Geometry check sheet. Reference: the model listing, model coordinates, mm. A direction names the side the tool comes from. Give positions to 0.01 mm unless a question says otherwise; leave off trailing zeros. Write each loop counter-clockwise with the first axis right and the second up, starting at its lowest first coordinate (ties: lowest second). Pieces come first, ordered by that corner, then holes. Notation, with made-up numbers: (40, 78.25) -> (87, 78.25) arc R5 ccw to (87, 83.25) -> close; hole circle Ø9 at (-5, 6). An arc over 180 degrees is marked (long way). One line per item, written item: value.
from build123d import *

# Parameters (mm, degrees)
BOSS_EXTRUDE1_DEPTH = 6.8
SKETCH2_W           = 3.55
SKETCH2_H           = 7.5
SKETCH2_W_2         = 2.085
SKETCH2_H_2         = 5
SKETCH2_H_3         = 8.5
CUT_EXTRUDE1_DEPTH  = 6.8
SKETCH3_R           = 6.1
CUT_EXTRUDE2_DEPTH  = 6.8
SKETCH4_R           = 1.75
CUT_EXTRUDE3_DEPTH  = 6.8


with BuildPart() as part:
    # Sketch1 → Boss-Extrude1 (new body)
    with BuildSketch(Plane.XY):
        with BuildLine():
            Line((-97, 195.4), (-92.5, 195.4))
            Line((-92.5, 195.4), (-92.5, 170.4))
            Line((-92.5, 170.4), (-89.2, 170.4))
            Line((-89.2, 170.4), (-89.2, 168.4))
            Line((-89.2, 168.4), (-82.3, 168.4))
            Line((-82.3, 168.4), (-82.3, 170.4))
            Line((-82.3, 170.4), (-79, 170.4))
            Line((-79, 170.4), (-79, 195.4))
            Line((-79, 195.4), (-75.034597787, 195.4))
            ThreePointArc((-75.034597787, 195.4), (-71.177872129, 193.996266659), (-69.125751269, 190.441889066))
            Line((-69.125751269, 190.441889066), (-64.181209637, 162.4))
            ThreePointArc((-64.181209637, 162.4), (-55.56310459, 141.196422986), (-39, 125.4))
            ThreePointArc((-39, 125.4), (-10.413345727, 95.649656796), (0, 55.726706578))
            Line((0, 55.726706578), (0, 0))
            Line((0, 0), (-78, 0))
            Line((-78, 0), (-78, 64.670637847))
            ThreePointArc((-78, 64.670637847), (-82.987756652, 97.72473667), (-97.652405773, 127.764697248))
            ThreePointArc((-97.652405773, 127.764697248), (-101.631906793, 135.904056195), (-103, 144.860278245))
            Line((-103, 144.860278245), (-103, 189.4))
            ThreePointArc((-103, 189.4), (-101.242640687, 193.642640687), (-97, 195.4))
        make_face()
    extrude(amount=BOSS_EXTRUDE1_DEPTH)

    # Sketch2 → Cut-Extrude1 (cut)
    with BuildSketch(Plane.XY.offset(6.8)):
        with Locations((-19, 17.25)):
            Rectangle(SKETCH2_W, SKETCH2_H)
        with Locations((-21.8175, 11)):
            Rectangle(SKETCH2_W_2, SKETCH2_H_2)
        with Locations((-16.1825, 11)):
            Rectangle(SKETCH2_W_2, SKETCH2_H_2)
        with Locations((-19, 4.25)):
            Rectangle(SKETCH2_W, SKETCH2_H_3)
        with Locations((-19, 11)):
            Rectangle(SKETCH2_W, SKETCH2_H_2)
    extrude(amount=-CUT_EXTRUDE1_DEPTH, mode=Mode.SUBTRACT)

    # Sketch3 → Cut-Extrude2 (cut)
    with BuildSketch(Plane.XY.offset(6.8)):
        with Locations((-59.04, -1.33811552)):
            Circle(SKETCH3_R)
    extrude(amount=-CUT_EXTRUDE2_DEPTH, mode=Mode.SUBTRACT)

    # Sketch4 → Cut-Extrude3 (cut)
    with BuildSketch(Plane(origin=(0, 0, 0), x_dir=(-1, 0, 0), z_dir=(0, 0, -1))):
        with Locations((64.000212357, 116.740381057)):
            Circle(SKETCH4_R)
        Polygon((84.488, 145.326270189), (78.512424714, 148.776270189), (74.512424714, 141.848066959), (80.488, 138.398066959), align=None)
        Polygon((63.488, 108.95320323), (57.512424714, 112.40320323), (53.512424714, 105.475), (59.488, 102.025), align=None)
    extrude(amount=-CUT_EXTRUDE3_DEPTH, mode=Mode.SUBTRACT)


solid = part.part
1) Depth check by flat-ended pin: pin 1 Ø1 at (x, z) = (-22, 4.5) entering from +Y; pin 2 Ø1 at (x, z) = (-16.5, 3) entering from +Y; pin 3 Ø1 at (x, y) = (-90, 110) entering from +Z; pin 4 Ø3.5 at (y, z) = (5, 3.5) entering from -X. Enter the tip coordinate at first touch or a pass-through.
Verdict:
pin 1: y = 112.05
pin 2: y = 105.63
pin 3: through
pin 4: x = -78
2) Sectioned sample at B-B on y = 136. Record the cut outline in (x, z).
Verdict:
outline: (-101.66, 0) -> (-51.55, 0) -> (-51.55, 6.8) -> (-101.66, 6.8) -> close
3) Tool access check on faces 5 (the flat face through (-92.5, 183, 3)), 6 (the flat face through (-20.775, 17, 3)), 7 (the flat face through (-61.46, 105.44, 3.35)). Record the directions out of +Z, -Z, +X, -X, +Y, -Y that give a thin tool (end or side, any length) a straight path to the whole face; none if there is none.
Verdict:
face 5: +Z, -Z, +Y
face 6: +Z, -Z, -Y
face 7: +Z, -Z
4) Sectioned sample at A-A on x = -11. Record the cut outline in (y, z), plus the area to 3 significant figures.
Verdict:
outline: (0, 0) -> (96.68, 0) -> (96.68, 6.8) -> (0, 6.8) -> close
area: 657 mm^2
5) Scan lines: probe 1 along X at (y, z) = (52, 4.5); probe 2 along X at (y, z) = (143.5, 3.5); probe 3 along X at (y, z) = (179, 1.5). Record each from-to range of solid material in increasing order.
Verdict:
probe 1: -78 to 0
probe 2: -102.97 to -83.43, -75.47 to -57.05
probe 3: -103 to -92.5, -79 to -67.11
6) Mould release check, pull along Y, two halves, no side actions. Record for faces 1 (the flat face through (-19, 21, 3)), 2 (the flat face through (-15.14, 11, 3)), 3 (the flat face through (-51, 77, 6.8)), 4 (the flat face through (-55.54, 108.99, 3.35)): released by +Y, released by -Y, zero draft, split by the parting line, or undercut.
Verdict:
face 1: released by -Y
face 2: undercut
face 3: zero draft
face 4: undercut
7) Sectioned sample at C-C on z = 2. Give the number of separate pieces and of enclosed holes in the cut face, plus the area to 3 significant figures.
Verdict:
separate pieces: 1
enclosed holes: 3
area: 11,600 mm^2
